from build123d import *

# Parameters (mm, degrees)
F0_W     = 101.6
F0_H     = 101.6
F0_W_2   = 76.2
F0_H_2   = 76.2
F1_DEPTH = 25.4
F2_W     = 76.2
F2_H     = 76.2
F6_D     = 19.05
F6_DEPTH = 76.2
F6_TIP   = 5.7231973962
F7_D     = 12.7
F7_DEPTH = 38.1
F7_TIP   = 3.8154649308


with BuildPart() as f1:
    # F0 (on Top) → F1 (new body)
    with BuildSketch(Plane.XY):
        with Locations((-1.3143327087, 25.9222988339)):
            Rectangle(F0_W, F0_H)
        with Locations((-1.3143327087, 25.9222988339)):
            Rectangle(F0_W_2, F0_H_2, mode=Mode.SUBTRACT)
        with Locations((-1.3143327087, 25.9222988339)):
            Rectangle(F0_W_2, F0_H_2)
    extrude(amount=F1_DEPTH)

    # F2 (on face) → F5 section 0
    with BuildSketch(Plane.XY.offset(25.4)):
        with Locations((-1.3143327087, 25.9222988339)):
            Rectangle(F2_W, F2_H)
    # F4 (on offset) → F5 section 1
    with BuildSketch(Plane.XY.offset(349.25)):
        Polygon((-1.3143327087, -9.9987256503), (34.6066917756, 25.9222988339), (-1.3143327087, 61.8433233182), (-37.235357193, 25.9222988339), align=None)
    loft()

    # F6
    with Locations(Plane(origin=(0, 0, 0), x_dir=(1, 0, 0), z_dir=(0, 0, -1))):
        with Locations((-1.3143327087, -25.9222988339)):
            Hole(F6_D / 2, depth=F6_DEPTH)
            with Locations((0, 0, -(F6_DEPTH + F6_TIP / 2))):  # 118° drill point
                Cone(0, F6_D / 2, F6_TIP, mode=Mode.SUBTRACT)

    # F7
    with Locations(Plane.XY.offset(349.25)):
        with Locations((-1.3143327087, 25.9222988339)):
            Hole(F7_D / 2, depth=F7_DEPTH)
            with Locations((0, 0, -(F7_DEPTH + F7_TIP / 2))):  # 118° drill point
                Cone(0, F7_D / 2, F7_TIP, mode=Mode.SUBTRACT)


solid = f1.part
Work out the finished part from the listing and answer in its coordinate system (mm). A direction names the side the tool comes from. Round coordinates to 2 decimals unless told otherwise and drop trailing zeros. Loops run counter-clockwise (first coordinate to the right, second up) from the corner with the lowest first, then second, coordinate; pieces in that order, holes last. Notation, with made-up numbers: (-24.75, -10) -> (32.25, -10) arc R22 ccw to (32.25, 3) -> close; hole circle Ø9 at (53.25, 1.5). An arc over 180 degrees is marked (long way). Use one line per item in the form item = value.
(1) Find section A-A on x = 43.5. Give the vertices of the cut face in (y, z), then the cut area to 3 significant figures.
Answer list:
outline = (-24.88, 0) -> (76.72, 0) -> (76.72, 25.4) -> (-24.88, 25.4) -> close
area = 2,580 mm2
(2) Flat-ended cylindrical pins translate along their axes: P1, Ø2, axis at y = 43.5, z = 256, coming from the +X side; P2, Ø8, axis at y = -12.5, z = 89.5, coming from the +X side; P3, Ø11.5, axis at x = -1.31, y = 25.92, coming from the +Z side. Find the tip coordinate at first contact, or state that the pin passes through.
Answer list:
P1 = 24.82
P2 = 29.79
P3 = 310.79
(3) A tool of negligible diameter and unlimited length cuts with its end or side. For faces 4 (the flat face through (-13, 27, 0)), 5 (the flat face through (43, 27, 25.4)), 6 (the cylindrical face through (-0.07, 16.48, 38.63)), from which of +Z, -Z, +X, -X, +Y, -Y can it reach the whole face along a straight path? Write none if from no direction.
Answer list:
face_4 = -Z, +X, -X, +Y, -Y
face_5 = +Z
face_6 = -Z
(4) For a pull along X with two mould halves and no side action, classify faces 1 (the flat face through (-2, 76.722, 13)), 2 (the flat face through (49.486, 25, 13)), 3 (the conical face through (-1.53, 24.28, 80.93)) as released by +X, released by -X, zero draft, split by the parting line, or undercut.
Answer list:
face_1 = zero draft
face_2 = released by +X
face_3 = undercut
(5) Straight lines are drawn through the part: line 1 (Z direction, x = -9.5, y = 68); line 2 (Y direction, x = -12.5, z = 181); line 3 (Y direction, x = 28, z = 330.5). For each, find the intervals that lie inside material, in ascending order.
Answer list:
line_1 = 0 to 25.4
line_2 = -1.73 to 60.36
line_3 = 20.52 to 34.08
